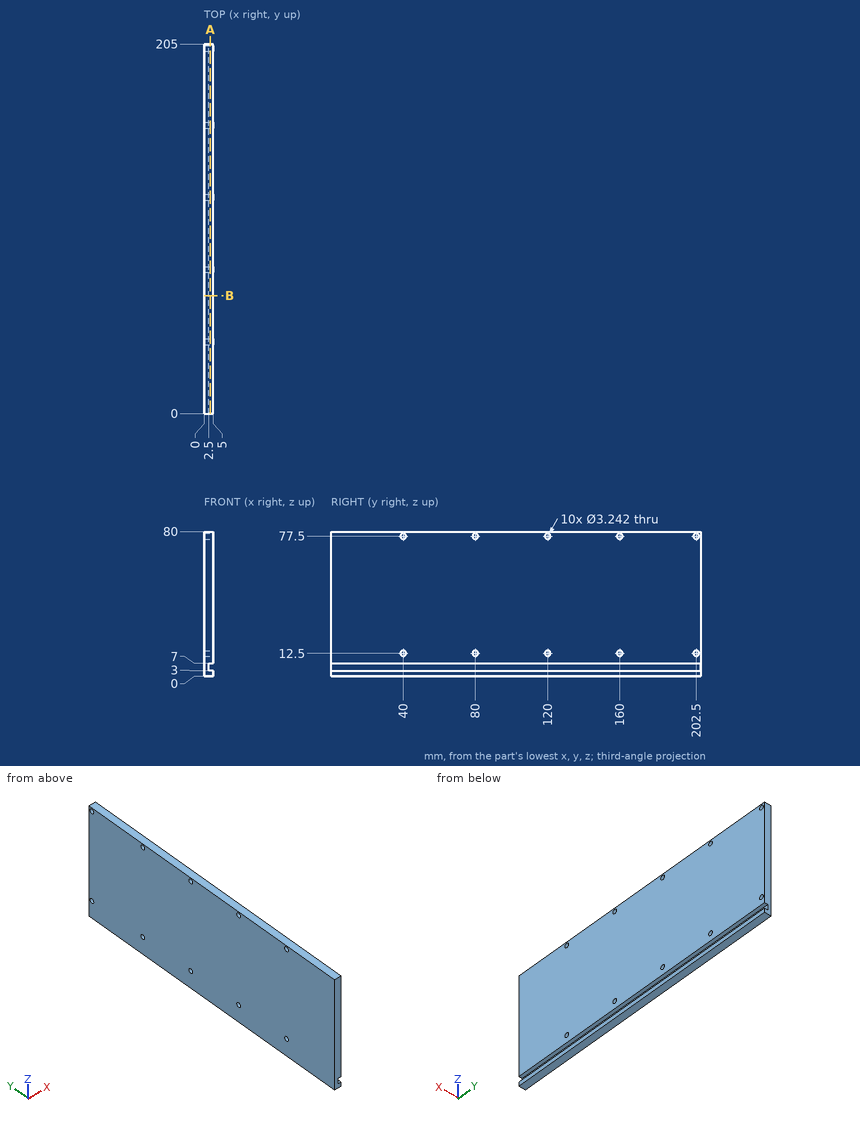
Geometry check sheet. Reference: drawing and pictorial views, mm from the part's lowest x, y, z. Coordinates: 2 decimals unless noted, no trailing zeros. Loops run counter-clockwise (first coordinate to the right, second up) from the corner with the lowest first, then second, coordinate; pieces in that order, holes last. Notation, with made-up numbers: M 71,-22.75 L 97,-22.75 A8 ccw 97,-15.75 Z; hole C 14,-36.75 d6. An arc over 180 degrees is marked long. One line per item, written item: value.
1. Section check A-A on x = 3.5. Give the number of separate pieces and of enclosed holes in the cut face, plus the area to 3 significant figures.
Answers follow:
separate pieces: 2
enclosed holes: 10
area: 15,500 mm^2
2. Material ranges on line 1 along Y through (x, z) = (2.5, 12.5); line 2 along Z through (x, y) = (4.05, 40); line 3 along Z through (x, y) = (4.65, 114.5), recorded low to high. Write a range as from..to.
Answers follow:
line 1: 0..38.38, 41.62..78.38, 81.62..118.38, 121.62..158.38, 161.62..200.88, 204.12..205
line 2: 0..3, 7..10.88, 14.12..75.88, 79.12..80
line 3: 0..3, 7..80
3. Section check B-B on y = 65.5. Record the cut outline in (x, z).
Answers follow:
outline: M 0,0 L 5,0 L 5,3 L 2.5,3 L 2.5,7 L 5,7 L 5,80 L 0,80 Z
